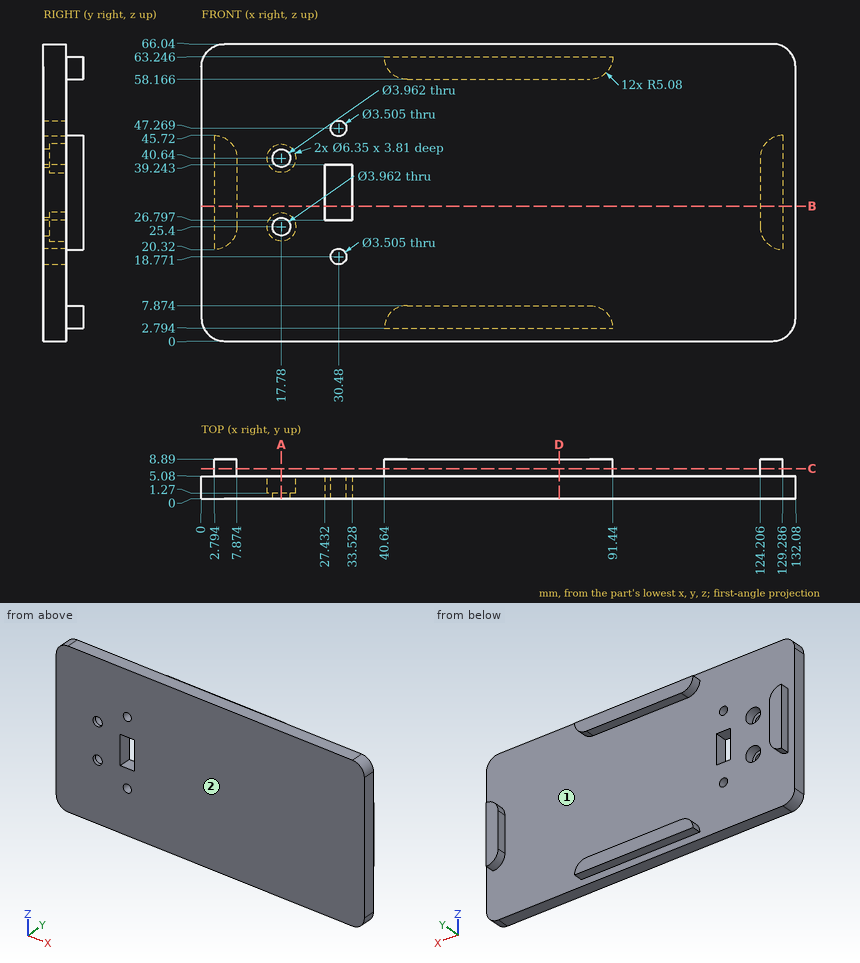
Input: dimensioned drawing with shaded views. Units: mm. Origin: part minimum x, y, z. Give positions to 0.01 mm unless a question says otherwise; leave off trailing zeros. Order: outer loops, then holes, each group sorted by start corner. A loop starts at its lowest first (then second) coordinate and runs counter-clockwise, first axis right, second up. Notation, with made-up numbers: (-11.75, 88) -> (24.25, 88) arc R21 ccw to (24.25, 95) -> close; hole circle Ø8 at (50, 41). An arc over 180 degrees is marked (long way). Write item = value, one per line.
Item 1: Section query B-B (z = 30). Output: boundary loops of the cut face in (x, y).
Check result:
outline = (0, 0) -> (27.43, 0) -> (27.43, 5.08) -> (7.87, 5.08) -> (7.87, 8.89) -> (2.79, 8.89) -> (2.79, 5.08) -> (0, 5.08) -> close; (33.53, 0) -> (132.08, 0) -> (132.08, 5.08) -> (129.29, 5.08) -> (129.29, 8.89) -> (124.21, 8.89) -> (124.21, 5.08) -> (33.53, 5.08) -> close
Item 2: Section query C-C (y = 6.75). State how many separate pieces and enclosed holes the cut face has, then the cut area to 3 significant figures.
Check result:
separate_pieces = 4
enclosed_holes = 0
area = 730 mm²
Item 3: Section query D-D (x = 79.5). Output: boundary loops of the cut face in (y, z).
Check result:
outline = (0, 0) -> (5.08, 0) -> (5.08, 2.79) -> (8.89, 2.79) -> (8.89, 7.87) -> (5.08, 7.87) -> (5.08, 58.17) -> (8.89, 58.17) -> (8.89, 63.25) -> (5.08, 63.25) -> (5.08, 66.04) -> (0, 66.04) -> close
Item 4: Mould query, pull axis X, two halves, no side actions, for the marked faces 1 and 2. Classes: +X half, -X half, draft (parallel to the pull), parting line (faces both ways), or undercut.
Check result:
face_1 = undercut
face_2 = draft
Item 5: Section query A-A (x = 17.78). Output: boundary loops of the cut face in (y, z) (1 decimal).
Check result:
outline = (0, 0) -> (5.1, 0) -> (5.1, 22.2) -> (1.3, 22.2) -> (1.3, 23.4) -> (0, 23.4) -> close; (0, 27.4) -> (1.3, 27.4) -> (1.3, 28.6) -> (5.1, 28.6) -> (5.1, 37.5) -> (1.3, 37.5) -> (1.3, 38.7) -> (0, 38.7) -> close; (0, 42.6) -> (1.3, 42.6) -> (1.3, 43.8) -> (5.1, 43.8) -> (5.1, 66) -> (0, 66) -> close
Item 6: Contact query for flat-ended pins moving along their axis: pin 1 (1.5 mm diameter, centred on x = 71, z = 22, fed in from +Y); pin 2 (1.9 mm diameter, centred on y = 7, z = 33.5, fed in from -X); pin 3 (1.9 mm diameter, centred on x = 64.5, y = 7, fed in from -Z). Output: stop coordinate, or through.
Check result:
pin_1 = 5.08
pin_2 = 2.79
pin_3 = 2.79
Item 7: Ray query, probe 1 along X at (y, z) = (4, 40.5); probe 2 along Z at (x, y) = (71, 8.5); probe 3 along X at (y, z) = (0.5, 25.4). Return the intervals inside material, ascending.
Check result:
probe_1 = 0 to 14.61, 20.95 to 132.08
probe_2 = 2.79 to 7.87, 58.17 to 63.25
probe_3 = 0 to 15.8, 19.76 to 132.08
